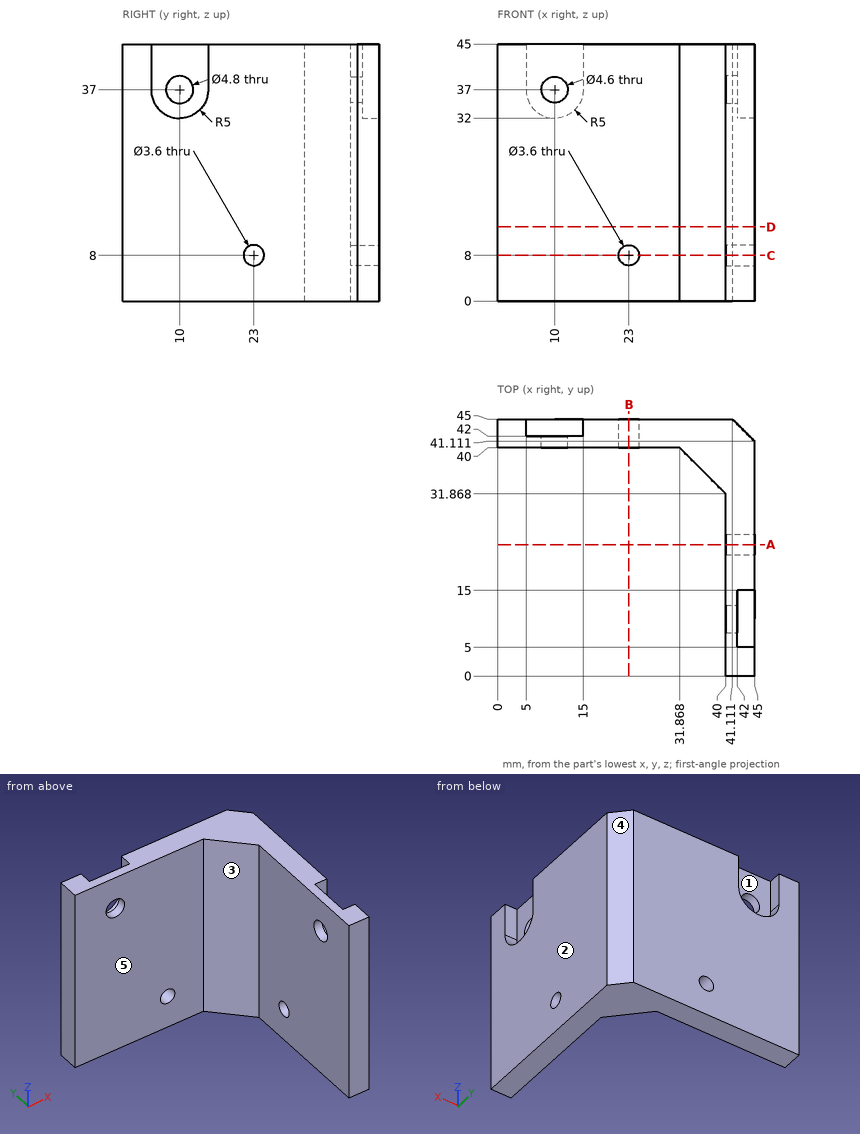
Geometry check sheet. Reference: drawing and pictorial views, mm from the part's lowest x, y, z. A direction names the side the tool comes from. Give positions to 0.01 mm unless a question says otherwise; leave off trailing zeros. Write each loop counter-clockwise with the first axis right and the second up, starting at its lowest first coordinate (ties: lowest second). Pieces come first, ordered by that corner, then holes. Notation, with made-up numbers: (-6.75, 34.5) -> (33.25, 34.5) arc R30 ccw to (33.25, 73.5) -> close; hole circle Ø6 at (-19, 51.25). An arc over 180 degrees is marked (long way). One line per item, written item: value. Start each with the question number.
Item 1: Material ranges on probe 1 along Z at (x, y) = (41.1, 23); probe 2 along X at (y, z) = (41.1, 37); probe 3 along Y at (x, z) = (20, 33), recorded low to high. Write a range as from..to.
Item 2: Section check D-D on z = 13. Record the cut outline in (x, y).
Item 3: Draft check along X on the marked faces 1, 2 and 3. Enter one of: +X half, -X half, draft (parallel to the pull), parting line (faces both ways), or undercut.
Item 4: Section check A-A on y = 23. Record the cut outline in (x, z), then the cut area to 3 significant figures.
Item 5: Section check C-C on z = 8. Record the cut outline in (x, y).
Item 6: Tool access check on the marked faces 4 and 5. Record the directions out of +Z, -Z, +X, -X, +Y, -Y that give a thin tool (end or side, any length) a straight path to the whole face; none if there is none.
Item 7: Gauge pin test, flat ends, axial feed: pin 1 (2.5 mm diameter, centred on y = 43, z = 41.5, fed in from +X); pin 2 (7.5 mm diameter, centred on y = 10, z = 37, fed in from +X); pin 3 (3 mm diameter, centred on x = 23, z = 8, fed in from -Y); pin 4 (5 mm diameter, centred on x = 9, z = 40.5, fed in from +Y). Record the tip position at first contact, or that the pin passes through.
Results list:
1. probe 1: 0..6.2, 9.8..45
1. probe 2: 0..7.7, 12.3..45
1. probe 3: 40..45
2. outline: (0, 40) -> (31.87, 40) -> (40, 31.87) -> (40, 0) -> (45, 0) -> (45, 41.11) -> (41.11, 45) -> (0, 45) -> close
3. face 1: undercut
3. face 2: +X half
3. face 3: -X half
4. outline: (40, 0) -> (45, 0) -> (45, 6.2) -> (40, 6.2) -> close; (40, 9.8) -> (45, 9.8) -> (45, 45) -> (40, 45) -> close
4. area: 207 mm²
5. outline: (0, 40) -> (21.2, 40) -> (21.2, 45) -> (0, 45) -> close; (24.8, 40) -> (31.87, 40) -> (40, 31.87) -> (40, 24.8) -> (45, 24.8) -> (45, 41.11) -> (41.11, 45) -> (24.8, 45) -> close; (40, 0) -> (45, 0) -> (45, 21.2) -> (40, 21.2) -> close
6. face 4: +Z, -Z, +X, +Y
6. face 5: +Z, -Z, -X, -Y
7. pin 1: x = 44.36
7. pin 2: x = 42
7. pin 3: through
7. pin 4: y = 42
